Geometry check sheet. Reference: the model listing, model coordinates, mm. A direction names the side the tool comes from. Round coordinates to 2 decimals unless told otherwise and drop trailing zeros. Write each loop counter-clockwise with the first axis right and the second up, starting at its lowest first coordinate (ties: lowest second). Pieces come first, ordered by that corner, then holes. Notation, with made-up numbers: M 32.5,-35.75 L 64.5,-35.75 A21 cw 64.5,-28.75 Z; hole C 60,-2.75 d8. An arc over 180 degrees is marked long. Use a Markdown table: item, result.
```python
from build123d import *

# Parameters (mm, degrees)
BOSS_EXTRUDE1_DEPTH = 31.88
FILLET1_R           = 0.5
SHELL1_T            = -1.5
SKETCH2_R           = 1.5
SKETCH2_R_2         = 0.6
BOSS_EXTRUDE2_DEPTH = 1.45


with BuildPart() as part:
    # Sketch1 → Boss-Extrude1 (new body)
    with BuildSketch(Plane(origin=(0, 0, 0), x_dir=(0, 0, -1), z_dir=(1, 0, 0))):
        Polygon((0, 0), (-7.85, 0), (-7.85, 3.15), (-1.5, 3.15), (-1.5, 9.6), (0, 9.6), align=None)
    extrude(amount=-BOSS_EXTRUDE1_DEPTH)

    # Fillet1
    fillet1_edges = [part.edges().sort_by_distance(p)[0] for p in [
        (0, 9.6, 0.75),
        (-31.88, 9.6, 0.75),
    ]]
    fillet(fillet1_edges, radius=FILLET1_R)

    # Shell1
    shell1_openings = [part.faces().sort_by_distance(p)[0] for p in [
        (-15.94, 0, 3.925),
    ]]
    offset(amount=SHELL1_T, openings=shell1_openings, kind=Kind.INTERSECTION)

    # Sketch2 → Boss-Extrude2 (add)
    # profile 1 of 3: a face of its own
    with BuildSketch(Plane.XZ.offset(-1.65)):
        with Locations(Location((-23.91, 3.925, 0), (0, 0, 90))):
            Circle(SKETCH2_R)
        with Locations(Location((-23.91, 3.925, 0), (0, 0, 270))):
            Circle(SKETCH2_R_2, mode=Mode.SUBTRACT)
    # profile 2 of 3: a face of its own
    with BuildSketch(Plane.XZ.offset(-1.65)):
        with Locations(Location((-15.94, 3.925, 0), (0, 0, 90))):
            Circle(SKETCH2_R)
        with Locations(Location((-15.94, 3.925, 0), (0, 0, 270))):
            Circle(SKETCH2_R_2, mode=Mode.SUBTRACT)
    # profile 3 of 3: a face of its own
    with BuildSketch(Plane.XZ.offset(-1.65)):
        with Locations(Location((-7.97, 3.925, 0), (0, 0, 90))):
            Circle(SKETCH2_R)
        with Locations(Location((-7.97, 3.925, 0), (0, 0, 270))):
            Circle(SKETCH2_R_2, mode=Mode.SUBTRACT)
    extrude(amount=BOSS_EXTRUDE2_DEPTH)


solid = part.part
```
Item 1: Go/stop test with flat-tipped pins: pin 1 (0.7 mm diameter, centred on x = -7.97, z = 3.925, fed in from +Y); pin 2 (1.3 mm diameter, centred on x = -16, z = 4, fed in from -Y); pin 3 (4 mm diameter, centred on x = -25, y = 6, fed in from +Z). Record where each tip stops, or that it passes through.
Outcome:
| item | result |
|---|---|
| pin 1 | stops at y = 3.15 |
| pin 2 | stops at y = 0.2 |
| pin 3 | stops at z = 1.5 |
Item 2: Cross-section at A-A, the plane y = 0.5. Record the cut outline in (x, z) (3 decimals).
Outcome:
| item | result |
|---|---|
| outline | M -31.88,0 L 0,0 L 0,7.85 L -31.88,7.85 Z; C -23.91,3.925 d3; C -15.94,3.925 d3; C -7.97,3.925 d3; hole M -30.38,1.5 L -1.5,1.5 L -1.5,6.35 L -30.38,6.35 Z; hole C -23.91,3.925 d1.2; hole C -15.94,3.925 d1.2; hole C -7.97,3.925 d1.2 |
Item 3: Access from +Z, -Z, +X, -X, +Y, -Y to the whole of each face (thin tool, end or side, straight path). Record for faces 4 (the face through (-16, 2, 7.85)), 5 (the face through (-15.345, 0.935, 4.003)).
Outcome:
| item | result |
|---|---|
| face 4 | +Z, +X, -X, +Y, -Y |
| face 5 | -Y |
Item 4: Cross-section at D-D, the plane x = -7.97. Record the cut outline in (y, z) (3 decimals).
Outcome:
| item | result |
|---|---|
| outline | M 0,0 L 9.6,0 L 9.6,1.5 L 3.15,1.5 L 3.15,7.85 L 0,7.85 L 0,6.35 L 1.65,6.35 L 1.65,5.425 L 0.2,5.425 L 0.2,4.525 L 1.65,4.525 L 1.65,3.325 L 0.2,3.325 L 0.2,2.425 L 1.65,2.425 L 1.65,1.5 L 0,1.5 Z |
Item 5: Cross-section at B-B, the plane x = -21. Record the cut outline in (y, z), and give its area (3 significant figures).
Outcome:
| item | result |
|---|---|
| outline | M 0,0 L 9.6,0 L 9.6,1.5 L 3.15,1.5 L 3.15,7.85 L 0,7.85 L 0,6.35 L 1.65,6.35 L 1.65,1.5 L 0,1.5 Z |
| area | 26.4 mm2 |
Item 6: Cross-section at C-C, the plane z = 6. Record the cut outline in (x, y), and give its area (3 significant figures).
Outcome:
| item | result |
|---|---|
| outline | M -31.88,0 L -30.38,0 L -30.38,1.65 L -1.5,1.65 L -1.5,0 L 0,0 L 0,3.15 L -31.88,3.15 Z |
| area | 52.8 mm2 |
Item 7: Mould release check, pull along Z, two halves, no side actions. Record for faces 1 (the face through (-16, 3.15, 5)), 2 (the face through (-23, 0.2, 4)), 3 (the face through (-16, 6, 1.5)): +Z half, -Z half, draft (parallel to the pull), parting line (faces both ways), or undercut.
Outcome:
| item | result |
|---|---|
| face 1 | draft |
| face 2 | undercut |
| face 3 | +Z half |
Item 8: Material ranges on line 1 along Z through (x, y) = (-26.5, 1.5); line 2 along Y through (x, z) = (-0.5, 4.75); line 3 along Y through (x, z) = (-15, 5), recorded low to high. Write a range as from..to.
Outcome:
| item | result |
|---|---|
| line 1 | z = 0..1.5, 6.35..7.85 |
| line 2 | y = 0..3.15 |
| line 3 | y = 0.2..3.15 |
